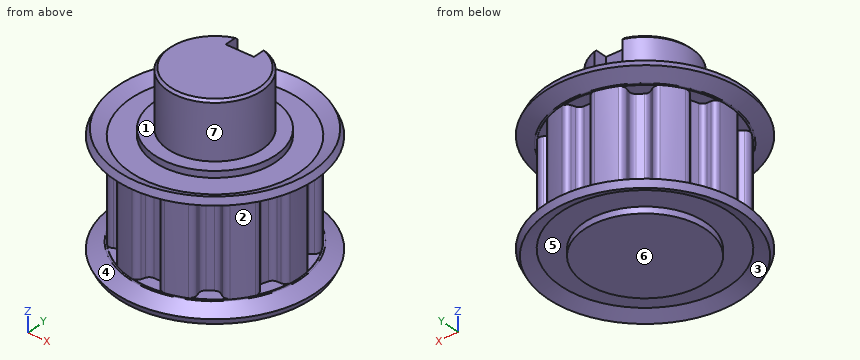
```python
from build123d import *

# Parameters (mm, degrees)
TOOTH_EXTRUDE_START      = -9.5
TOOTH_EXTRUDE_DEPTH      = 19
PATTERN_CIRCULAR_1_COUNT = 10
SKETCH_3_R               = 10
EXTRUDE_1_DEPTH          = 12
CHAMFER_1_SIZE           = 0.5
SKETCH_4_W               = 6
SKETCH_4_H               = 7
CUT_EXTRUDE_1_DEPTH      = 12
FILLET_1_R               = 3


with BuildPart() as part:
    # GearBelt-BaseSketch → 0.375in Pitch 'L', 0.500in Belt Width, 36.3828mm P.D. (revolve)
    with BuildSketch(Plane(origin=(0, 0, 0), x_dir=(0, 0, -1), z_dir=(1, 0, 0)), mode=Mode.PRIVATE) as f_0_375in_pitch_l_0_500in_belt_width_36_sk:
        Polygon((-12.5, 0), (12.5, 0), (12.5, 12.857409477), (11.136655608, 12.857409477), (11.136655608, 17.838520326), (12.5, 20.614224723), (11.136655777, 21.283859322), (9.617735592, 18.191410003), (9.617735592, 17.810409995), (-9.617735592, 17.810409995), (-9.617735592, 18.191410003), (-11.136655777, 21.283859322), (-12.5, 20.614224723), (-11.136655608, 17.838520326), (-11.136655608, 12.857409477), (-12.5, 12.857409477), align=None)
    revolve(f_0_375in_pitch_l_0_500in_belt_width_36_sk.sketch.rotate(Axis((0, 0, 14.2875), (0, 0, -1)), 90), axis=Axis((0, 0, 14.2875), (0, 0, -1)))

    # Tooth-Sketch → Tooth-Extrude (cut)
    with BuildSketch(Plane.XY.offset(TOOTH_EXTRUDE_START)):
        with BuildLine():
            Line((-0.690315485, 15.14340994), (0.690315485, 15.14340994))
            ThreePointArc((0.690315485, 15.14340994), (1.373229902, 15.358732029), (1.809136966, 15.926817177))
            Line((1.809136966, 15.926817177), (2.101875716, 16.731110287))
            ThreePointArc((2.101875716, 16.731110287), (2.625223607, 17.348846453), (3.424464642, 17.478093321))
            Line((3.424464642, 17.478093321), (3.424464642, 20.018093321))
            Line((3.424464642, 20.018093321), (-3.424464642, 20.018093321))
            Line((-3.424464642, 20.018093321), (-3.424464642, 17.478093321))
            ThreePointArc((-3.424464642, 17.478093321), (-2.625223607, 17.348846453), (-2.101875716, 16.731110287))
            Line((-2.101875716, 16.731110287), (-1.809136966, 15.926817177))
            ThreePointArc((-1.809136966, 15.926817177), (-1.373229902, 15.358732029), (-0.690315485, 15.14340994))
        make_face()
    tooth_extrude = extrude(amount=TOOTH_EXTRUDE_DEPTH, mode=Mode.SUBTRACT)

    # 阵列(圆周)1: Tooth-Extrude ×10 about axis
    pattern_circular_1_axis = Axis((0, 0, 0), (0, 0, 1))
    for i in range(1, PATTERN_CIRCULAR_1_COUNT):
        add(tooth_extrude.rotate(pattern_circular_1_axis, i * 360 / PATTERN_CIRCULAR_1_COUNT), mode=Mode.SUBTRACT)

    # 草图3 → 凸台-拉伸1 (add)
    with BuildSketch(Plane.XY.offset(12.5)):
        with Locations(Location((0, 0, 0), (0, 0, 180))):
            Circle(SKETCH_3_R)
    extrude(amount=EXTRUDE_1_DEPTH)

    # 倒角1
    chamfer_1_edges = [part.edges().sort_by_distance(p)[0] for p in [
        (10, 0, 24.5),
    ]]
    chamfer(chamfer_1_edges, length=CHAMFER_1_SIZE)

    # 草图4 → 切除-拉伸1 (cut)
    with BuildSketch(Plane.XY.offset(24.5)):
        with Locations((0, 10)):
            Rectangle(SKETCH_4_W, SKETCH_4_H)
    extrude(amount=-CUT_EXTRUDE_1_DEPTH, mode=Mode.SUBTRACT)

    # 圆角1
    fillet_1_edges = [part.edges().sort_by_distance(p)[0] for p in [
        (-3, 8.019696007, 12.5),
        (3, 8.019696007, 12.5),
    ]]
    fillet(fillet_1_edges, radius=FILLET_1_R - 0.0001)  # a hair under: the kernel refuses the full size


solid = part.part
```
Design review of the part built by this model. Coordinates are the model's own, in mm. Face numbers are marked on the shaded views. A direction names the side the tool comes from. Give positions to 0.01 mm unless a question says otherwise; leave off trailing zeros. Write item = value, one per line. Start each with the question number.
(1) For the marked faces 4, 5, 6 and 7, list the 3-axis set-ups (+Z, -Z, +X, -X, +Y, -Y) from which the entire face can be reached by the end or side of a thin tool; tool diameter is ignored.
(2) To check wall thickness, follow line 1 along Z through (x, y) = (10.5, -8.5); line 2 along X through (y, z) = (16, 4.5); line 3 along X through (y, z) = (12, 3). State the ranges of each line that lie inside material, in increasing order.
(3) For pin 1 (1.3 mm diameter, centred on x = -0.5, y = 16.5, fed in from -Z); pin 2 (10 mm diameter, centred on y = 9.5, z = 16, fed in from +X); pin 3 (2.5 mm diameter, centred on x = 10, y = -13.5, fed in from -Z), all flat-tipped, find the tip position at first contact; note any pin that passes through.
(4) Mouldability with a two-part tool opening along Z and no side actions: class the marked faces 1, 2 and 3 as +Z half, -Z half, draft (parallel to the pull), parting line (faces both ways), or undercut.
Numbers:
q1.face_4 = none
q1.face_5 = -Z
q1.face_6 = -Z, +X, -X, +Y, -Y
q1.face_7 = +Z
q2.line_1 = -11.14 to 11.14
q2.line_2 = -7.75 to -1.84, 1.84 to 7.75
q2.line_3 = -13.16 to -11.09, -9.25 to 9.25, 11.09 to 13.16
q3.pin_1 = -11.14
q3.pin_2 = 19.83
q3.pin_3 = -11.24
q4.face_1 = +Z half
q4.face_2 = undercut
q4.face_3 = -Z half
